from build123d import *

# Parameters (mm, degrees)
F1_DEPTH      = 2
F2_DEPTH      = 8
F3_T          = 1
F3_T3_DEPTH   = 101
F3_T6_ANGLE   = 180.000000001
F3_T8_ANGLE   = 180.000000001
F7_DEPTH      = 25
F7_DEPTH_BACK = 25


# Not quite as in the source:
# - a shell that OpenCascade refuses in one call is made with other operations: the cavity is built on its own and cut out


with BuildPart() as f1:
    # F0 (on Top) → F1 (new body)
    with BuildSketch(Plane.XY):
        with BuildLine():
            Line((0, 19.999999553), (-99, 19.999999553))
            ThreePointArc((-99, 19.999999553), (-118.999999553, 0), (-99, -19.999999553))
            Line((-99, -19.999999553), (0, -19.999999553))
            ThreePointArc((0, -19.999999553), (19.999999553, 0), (0, 19.999999553))
        make_face()
        with BuildLine():
            ThreePointArc((0, 15), (15, 0), (0, -15))
            Line((0, -15), (-99, -15))
            ThreePointArc((-99, -15), (-114, 0), (-99, 15))
            Line((-99, 15), (0, 15))
        make_face(mode=Mode.SUBTRACT)
        with BuildLine():
            Line((-99, -15), (0, -15))
            ThreePointArc((0, -15), (15, 0), (0, 15))
            Line((0, 15), (-99, 15))
            ThreePointArc((-99, 15), (-114, 0), (-99, -15))
        make_face()
    extrude(amount=-F1_DEPTH)

    # F0 (on Top) → F2 (join)
    with BuildSketch(Plane.XY):
        with BuildLine():
            Line((-99, -15), (0, -15))
            ThreePointArc((0, -15), (15, 0), (0, 15))
            Line((0, 15), (-99, 15))
            ThreePointArc((-99, 15), (-114, 0), (-99, -15))
        make_face()
    extrude(amount=F2_DEPTH)

    # F3: shell of thickness 1, made by hand


with BuildPart() as f3_core1:
    # F3_t2: copy of F1
    add(f1.part)

    # the walls: a layer under each face that stays
    f3_faces = [f3_core1.faces().sort_by_distance(p)[0] for p in [
        (-49.5, -19.999999553, -1),
        (-118.999999553, 0, -1),
        (19.999999553, 0, -1),
        (-109.0714281883, -17.1428567597, 0),
        (-49.5, 0, -2),
        (-49.5, 19.999999553, -1),
        (-49.5, -15, 4),
        (15, 0, 4),
        (-49.5, 15, 4),
        (-114, 0, 4),
    ]]
    thicken(f3_faces, amount=-F3_T, mode=Mode.SUBTRACT)

    # F3_s4 → F3_t3 (cut)
    with BuildSketch(Plane.YZ.offset(-100)):
        Polygon((-15.01, 0.01), (-15, -1), (-14, -1), (-14, 0), align=None)
        Polygon((15.01, 0.01), (15, -1), (14, -1), (14, 0), align=None)
    extrude(amount=F3_T3_DEPTH, mode=Mode.SUBTRACT)

    # F3_s5 → F3_t6 (revolve, cut)
    with BuildSketch(Plane.YZ):
        Polygon((-15.01, 0.01), (-15, -1), (-14, -1), (-14, 0), align=None)
    revolve(axis=Axis((0, 0, 0), (0, 0, 1)), revolution_arc=F3_T6_ANGLE, mode=Mode.SUBTRACT)

    # F3_s7 → F3_t8 (revolve, cut)
    with BuildSketch(Plane.YZ.offset(-99)):
        Polygon((15.01, 0.01), (15, -1), (14, -1), (14, 0), align=None)
    revolve(axis=Axis((-99, 0, 0), (0, 0, 1)), revolution_arc=F3_T8_ANGLE, mode=Mode.SUBTRACT)


with BuildPart() as f1_1:
    add(f1.part)

    # what is left inside the walls is the cavity
    f3_cavity = [f3_core1.part.solids().sort_by_distance(p)[0] for p in [
        (-49.5, -4.666667, 7.99),
    ]]
    add(f3_cavity, mode=Mode.SUBTRACT)

    # F5: sweep along a path in F5_path
    with BuildLine(Plane(origin=(0, 15, 8), x_dir=(0, -1, 0), z_dir=(0, 0, -1))) as f5_path:
        Line((0, 0), (0, 99))
    # F4 (on Right) → F5 (sweep)
    with BuildSketch(Plane.YZ):
        Polygon((16, 5.01), (15, 8), (15, 5.01), align=None)
        Polygon((-15, 5.01), (-15, 8), (-16, 5.01), align=None)
    sweep(path=f5_path.line)

    # F6 (on Front) → F7 (cut, two sides)
    with BuildSketch(Plane.XZ) as f7_sk:
        with BuildLine():
            ThreePointArc((-100.2408070591, 3.0141202733), (-99.000737071, 1.7740502852), (-97.760667083, 3.0141202733))
            Line((-97.760667083, 3.0141202733), (-97.760667083, 9.1903032735))
            Line((-97.760667083, 9.1903032735), (-100.2408070591, 9.8686125129))
            Line((-100.2408070591, 9.8686125129), (-100.2408070591, 3.0141202733))
        make_face()
        with BuildLine():
            Line((-1.2400699881, 9.1903032735), (-1.2400699881, 3.0141202733))
            ThreePointArc((-1.2400699881, 3.0141202733), (0, 1.7740502852), (1.2400699881, 3.0141202733))
            Line((1.2400699881, 3.0141202733), (1.2400699881, 9.8686125129))
            Line((1.2400699881, 9.8686125129), (-1.2400699881, 9.1903032735))
        make_face()
    extrude(amount=-F7_DEPTH, mode=Mode.SUBTRACT)
    extrude(f7_sk.sketch, amount=F7_DEPTH_BACK, mode=Mode.SUBTRACT)


solid = f1_1.part
Work out the finished part from the listing and answer in its coordinate system (mm). A direction names the side the tool comes from. Round coordinates to 2 decimals unless told otherwise and drop trailing zeros. Loops run counter-clockwise (first coordinate to the right, second up) from the corner with the lowest first, then second, coordinate; pieces in that order, holes last. Notation, with made-up numbers: (-19, 18) -> (-12, 18) arc R26 ccw to (-12, 36) -> close; hole circle Ø1 at (27, -13.75). An arc over 180 degrees is marked (long way). Use one line per item in the form item = value.
(1) For a pull along Z with two mould halves and no side action, classify faces 1 (the flat face through (-49, 15, 2)), 2 (the flat face through (-50, 14, 3)), 3 (the flat face through (-113.3, 0.1, 8)) as released by +Z, released by -Z, zero draft, split by the parting line, or undercut.
Answer list:
face_1 = undercut
face_2 = zero draft
face_3 = released by +Z
(2) A tool of negligible diameter and unlimited length cuts with its end or side. For faces 4 (the cylindrical face through (-114, 0, 4)), 5 (the cylindrical face through (-113, 0, 3)), 6 (the flat face through (-50, -15, 2)), 7 (the cylindrical face through (15, 0, 4)), from which of +Z, -Z, +X, -X, +Y, -Y can it reach the whole face along a straight path? Write none if from no direction.
Answer list:
face_4 = +Z, -X
face_5 = +Z
face_6 = +X, -X, -Y
face_7 = +Z, +X
(3) Straight lines are drawn through the part: line 1 (Y direction, x = -14, z = 2); line 2 (Y direction, x = -11, z = -0.5); line 3 (Z direction, x = -31, y = 7). For each, find the intervals that lie inside material, in ascending order.
Answer list:
line_1 = -15 to -14, 14 to 15
line_2 = -20 to -14, 14 to 20
line_3 = -2 to -1
(4) Find section C-C on y = -9.5. Give the vertices of the cut face in (x, z), then the cut area to 3 significant figures.
Answer list:
outline = (-116.6, -2) -> (17.6, -2) -> (17.6, 0) -> (11.61, 0) -> (11.61, 8) -> (10.28, 8) -> (10.28, -1) -> (-109.28, -1) -> (-109.28, 8) -> (-110.61, 8) -> (-110.61, 0) -> (-116.6, 0) -> close
area = 170 mm2
(5) Find section A-A on x = -15. Give the vertices of the cut face in (y, z), then the cut area to 3 significant figures.
Answer list:
outline = (-20, -2) -> (20, -2) -> (20, 0) -> (15, 0) -> (15, 5.01) -> (16, 5.01) -> (15, 8) -> (14, 8) -> (14, -1) -> (-14, -1) -> (-14, 8) -> (-15, 8) -> (-16, 5.01) -> (-15, 5.01) -> (-15, 0) -> (-20, 0) -> close
area = 71.0 mm2
(6) Flat-ended cylindrical pins translate along their axes: P1, Ø2.5, axis at x = -37, z = 1.5, coming from the +Y side; P2, Ø12, axis at x = -29.5, y = -1, coming from the +Z side; P3, Ø1.1, axis at y = -14, z = 6.5, coming from the +X side; P4, Ø20, axis at x = -76.5, y = -8.5, coming from the +Z side. Find the tip coordinate at first contact, or state that the pin passes through.
Answer list:
P1 = 15
P2 = -1
P3 = 6.64
P4 = 8
(7) Find section B-B on y = 0. Give the vertices of the cut face in (x, z), then the cut area to 3 significant figures.
Answer list:
outline = (-119, -2) -> (20, -2) -> (20, 0) -> (15, 0) -> (15, 8) -> (14, 8) -> (14, -1) -> (-113, -1) -> (-113, 8) -> (-114, 8) -> (-114, 0) -> (-119, 0) -> close
area = 167 mm2
